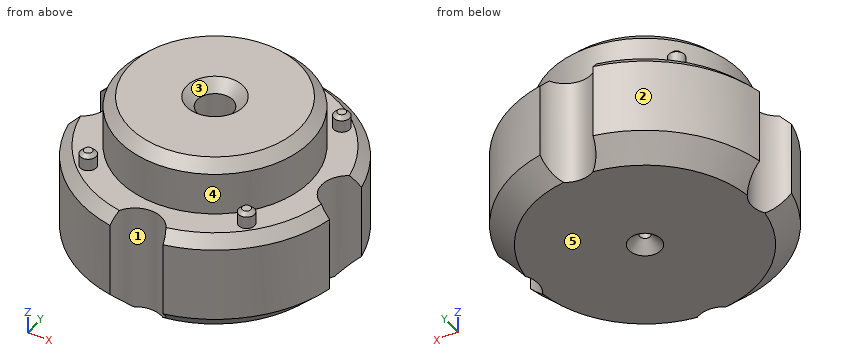
Autodesk Inventor part; units mm, degrees
ref_plane "YZ Plane" through (0, 0, 0) normal (1, 0, 0) x (0, 1, 0)
ref_plane "XZ Plane" through (0, 0, 0) normal (0, 1, 0) x (-1, 0, 0)
ref_plane "XY Plane" through (0, 0, 0) normal (0, 0, 1) x (1, 0, 0)
sketch "Sketch1" plane through (0, 0, 0) normal (0, 0, 1) x (1, 0, 0)
  circle A0 centre (0, 0) radius 12.5
  dimension "d0" = 25
extrude "Extrusion1" add sketch "Sketch1" along normal blind 15
chamfer "Chamfer2" distance 2 angle 45 1 edges at (-12.5, 0, 0)
sketch "Sketch2" plane through (0, 0, 0) normal (1, 0, 0) x (0, 1, 0)
  line L0 (0, 0) -> (0.5, 0)
  line L1 (0.5, 0) -> (0.5, 4)
  line L2 (0.5, 4) -> (0, 4)
  line L3 (0, 4) -> (0, 0)
  line L4 (12.5, 15) -> (-12.5, 15)
  line L5 (0, 4) -> (1.675, 4)
  line L6 (1.675, 4) -> (1.675, 15)
  line L7 (1.675, 15) -> (0, 15)
  line L8 (0, 15) -> (0, 4)
  dimension "d9" = 0.5
  dimension "d10" = 1.675
  dimension "d11" = 4
revolve "Revolution1" cut sketch "Sketch2" angle 360 about axis through (0, 0, 15) along (0, 0, -1)
chamfer "Chamfer3" distance 1 angle 45 2 edges at (0, -0.5, 0) (0, -1.675, 15)
sketch "Sketch3" plane through (0, 0, 15) normal (0, 0, 1) x (1, 0, 0)
  circle A0 centre (0, 0) radius 9
  circle A1 centre (0, 0) radius 0.5 construction
  line L0 (0, 0) -> (26.029, 0) construction
  circle A2 centre (0, 0) radius 12.5 construction
  circle A3 centre (12.5, 0) radius 2.5
  circle A4 centre (0, 12.5) radius 2.5
  circle A5 centre (-12.5, 0) radius 2.5
  circle A6 centre (0, -12.5) radius 2.5
  circle A7 centre (0, 0) radius 12.5
  point P0 (-2.4875, 12.25)
  point P1 (-12.25, 2.4875)
  point P2 (-12.25, -2.4875)
  point P3 (-2.4875, -12.25)
  point P4 (2.4875, -12.25)
  point P5 (12.25, -2.4875)
  point P6 (12.25, 2.4875)
  point P7 (2.4875, 12.25)
  dimension "d16" = 5
  dimension "d19" = 360
  dimension "d21" = 25
  dimension "d22" = 18
extrude "Extrusion2" cut sketch "Sketch3" against normal through all contours A3 A7 | A7 A3 | A7 A4 | A4 A7 | A7 A6 | A6 A7 | A7 A5 | A5 A7
extrude "Extrusion3" cut sketch "Sketch3" against normal blind 5 contours A3 A7 A6 A5 A4
chamfer "Chamfer4" distance 1 angle 45 5 edges at (-9, 0, 15) (-8.8388, -8.8388, 10) (8.8388, -8.8388, 10) (8.8388, 8.8388, 10) (-8.8388, 8.8388, 10)
sketch "Sketch4" plane through (0, 0, 10) normal (0, 0, 1) x (1, 0, 0)
  circle A0 centre (0, 0) radius 0.5 construction
  line L0 (0, 0) -> (-18.6595, 0) construction
  line L1 (0, 0) -> (0, 25.4609) construction
  circle A1 centre (0, 0) radius 1.675 construction
  line L2 (0, 0) -> (-16.5294, 16.5294) construction
  circle A2 centre (-7.4246, 7.4246) radius 0.75
  circle A3 centre (0, 0) radius 2.675 construction
  circle A4 centre (0, 0) radius 10.5 construction
  circle A5 centre (-7.4246, -7.4246) radius 0.75
  circle A6 centre (7.4246, -7.4246) radius 0.75
  circle A7 centre (7.4246, 7.4246) radius 0.75
  point P0 (0, 0)
  dimension "d31" = 21
  dimension "d30" = 45
  dimension "d32" = 1.5
  dimension "d35" = 360
extrude "Extrusion4" add sketch "Sketch4" along normal blind 1.5
chamfer "Chamfer5" distance 0.35 angle 45 4 edges at (6.6746, 7.4246, 11.5) (-8.1746, 7.4246, 11.5) (-8.1746, -7.4246, 11.5) (6.6746, -7.4246, 11.5)
properties part number "centrifugetool_3.2mm_base_v3"
Can you work these out from the model? Positions are in its coordinate system, mm. Face numbers are marked on the shaded views. A direction names the side the tool comes from. Round coordinates to 2 decimals unless told otherwise and drop trailing zeros. Loops run counter-clockwise (first coordinate to the right, second up) from the corner with the lowest first, then second, coordinate; pieces in that order, holes last. Notation, with made-up numbers: (55, 79.5) -> (73, 79.5) arc R10 cw to (73, 95.5) -> close; hole circle Ø11 at (-12, 11.25). An arc over 180 degrees is marked (long way). Answer in a Markdown table with one row per item.
Item 1: Suppose I cut it at D-D, the plane z = 10.5. List the corners of the cut face in (x, y) for me (3 decimals).
Answer block:
| item | result |
|---|---|
| outline | circle Ø18 at (0, 0); circle Ø1.5 at (-7.425, -7.425); circle Ø1.5 at (-7.425, 7.425); circle Ø1.5 at (7.425, -7.425); circle Ø1.5 at (7.425, 7.425); hole circle Ø3.35 at (0, 0) |
Item 2: Will these pins go through, and if not, where does the flat tip stop? P1, Ø0.6, axis at x = -7.5, y = -7.5, coming from the +Z side; P2, Ø4.5, axis at x = 0, y = 0, coming from the +Z side (3 decimals); P3, Ø1.5, axis at y = -1, z = 6.5, coming from the +X side.
Answer block:
| item | result |
|---|---|
| P1 | z = 11.5 |
| P2 | z = 14.575 |
| P3 | x = 10.71 |
Item 3: Suppose I cut it at A-A, the plane x = 0. List the corners of the cut face in (y, z) for me (3 decimals).
Answer block:
| item | result |
|---|---|
| outline | (-10, 0) -> (-1.5, 0) -> (-0.5, 1) -> (-0.5, 4) -> (-1.675, 4) -> (-1.675, 14) -> (-2.675, 15) -> (-8, 15) -> (-9, 14) -> (-9, 10) -> (-10, 10) -> close; (0.5, 1) -> (1.5, 0) -> (10, 0) -> (10, 10) -> (9, 10) -> (9, 14) -> (8, 15) -> (2.675, 15) -> (1.675, 14) -> (1.675, 4) -> (0.5, 4) -> close |
Item 4: We'd pull the mould along Y, two halves only. Please class the marked faces 1, 2 and 3: released by +Y, released by -Y, zero draft, split by the parting line, or undercut.
Answer block:
| item | result |
|---|---|
| face 1 | released by -Y |
| face 2 | released by +Y |
| face 3 | undercut |
Item 5: If I drill on probe 1 along X at (y, z) = (0, 8) (3 decimals); probe 2 along Y at (x, z) = (10.25, 1); probe 3 along Y at (x, z) = (-0.75, 5.5), over which ranges is the centre line in solid material (lowest first)?
Answer block:
| item | result |
|---|---|
| probe 1 | -10 to -1.675, 1.675 to 10 |
| probe 2 | -5.21 to -1.09, 1.09 to 5.21 |
| probe 3 | -10.12 to -1.5, 1.5 to 10.12 |
Item 6: Suppose I cut it at B-B, the plane z = 6. List the corners of the cut face in (x, y) for me (3 decimals).
Answer block:
| item | result |
|---|---|
| outline | (-12.25, -2.487) arc R12.5 ccw to (-2.487, -12.25) arc R2.5 cw to (2.487, -12.25) arc R12.5 ccw to (12.25, -2.487) arc R2.5 cw to (12.25, 2.487) arc R12.5 ccw to (2.487, 12.25) arc R2.5 cw to (-2.487, 12.25) arc R12.5 ccw to (-12.25, 2.487) arc R2.5 cw to start; hole circle Ø3.35 at (0, 0) |
Item 7: On a 3-axis mill with a long thin cutter (end or side, diameter ignored), from which of +Z, -Z, +X, -X, +Y, -Y can I reach the whole of each face in a straight line? I mean the marked faces 4 and 5. Say none if no direction works.
Answer block:
| item | result |
|---|---|
| face 4 | +Z |
| face 5 | -Z, +X, -X, +Y, -Y |
